from build123d import *

# Parameters (mm, degrees)
F0_R     = 50
F1_DEPTH = 50
F2_R     = 12.5
F3_DEPTH = 104.2
F4_R     = 44.950947
F5_DEPTH = 45.9


with BuildPart() as f1:
    # F0 (on Front) → F1 (new body)
    with BuildSketch(Plane.XZ):
        Circle(F0_R)
    extrude(amount=-F1_DEPTH)

    # F2 (on Top) → F3 (cut, symmetric)
    with BuildSketch(Plane.XY):
        with Locations((0, 29.318675)):
            Circle(F2_R)
    extrude(amount=F3_DEPTH, both=True, mode=Mode.SUBTRACT)

    # F4 (on Front) → F5 (cut)
    with BuildSketch(Plane.XZ):
        Circle(F4_R)
    extrude(amount=-F5_DEPTH, mode=Mode.SUBTRACT)


solid = f1.part
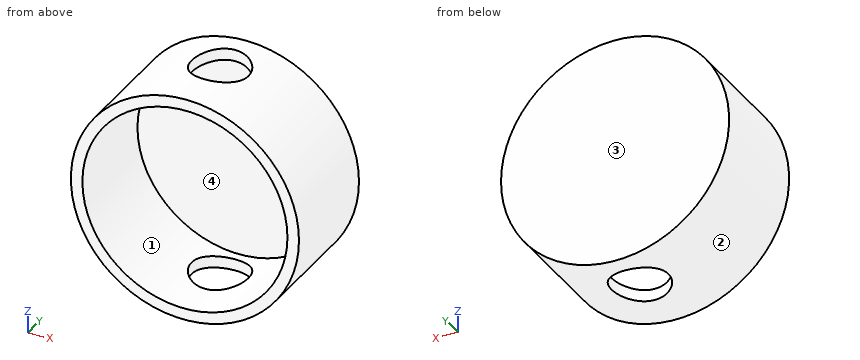
Geometry: final body of the model. Coordinates: model frame, mm. Face numbers are marked on the shaded views. Round coordinates to 2 decimals unless told otherwise and drop trailing zeros. Loops run counter-clockwise (first coordinate to the right, second up) from the corner with the lowest first, then second, coordinate; pieces in that order, holes last. Notation, with made-up numbers: M 86,-15.5 L 120,-15.5 A21 cw 120,-11.5 Z; hole C 54.25,-32.75 d10. An arc over 180 degrees is marked long. One line per question, with ' | ' between items.
(1) Material intervals for line 1 along Y through (x, z) = (0, -46.5); line 2 along Y through (x, z) = (0, -44.75); line 3 along X through (y, z) = (34.5, 15.5), sorted ascending. Write a range as from..to.
Check result:
line 1: y = 0..16.82, 41.82..50 | line 2: y = 45.9..50 | line 3: x = -47.54..-42.19, 42.19..47.54
(2) Cut plane A-A on x = 0. Return the cut outline in (y, z), plus the area to 3 significant figures.
Check result:
outline: M 0,-50 L 16.82,-50 L 16.82,-44.95 L 0,-44.95 Z; M 0,44.95 L 16.82,44.95 L 16.82,50 L 0,50 Z; M 41.82,-50 L 50,-50 L 50,50 L 41.82,50 L 41.82,44.95 L 45.9,44.95 L 45.9,-44.95 L 41.82,-44.95 Z | area: 621 mm2
(3) Cut plane C-C on x = 35. Return the cut outline in (y, z), plus the area to 3 significant figures.
Check result:
outline: M 0,-35.71 L 50,-35.71 L 50,35.71 L 0,35.71 L 0,28.21 L 45.9,28.21 L 45.9,-28.21 L 0,-28.21 Z | area: 981 mm2
(4) Contact query for flat-ended pins moving along their axis: P1, Ø5, axis at y = 15, z = -24.5, coming from the +X side; P2, Ø2, axis at x = 15.5, y = 17.5, coming from the -Z side; P3, Ø1, axis at x = -11.5, y = 38.5, coming from the +Z side (3 decimals). Output: stop coordinate, or through.
Check result:
P1: stops at x = 44.9 | P2: stops at z = -47.85 | P3: stops at z = 48.775
(5) Cut plane B-B on z = 0. Return the cut outline in (x, y), plus the area to 3 significant figures.
Check result:
outline: M -50,0 L -44.95,0 L -44.95,45.9 L 44.95,45.9 L 44.95,0 L 50,0 L 50,50 L -50,50 Z | area: 874 mm2
(6) Pull-direction query (Z, two-part tool) for the marked faces 1, 2, 3 and 4; classes: +Z half, -Z half, draft (parallel to the pull), parting line (faces both ways), or undercut.
Check result:
face 1: undercut | face 2: parting line | face 3: draft | face 4: undercut
